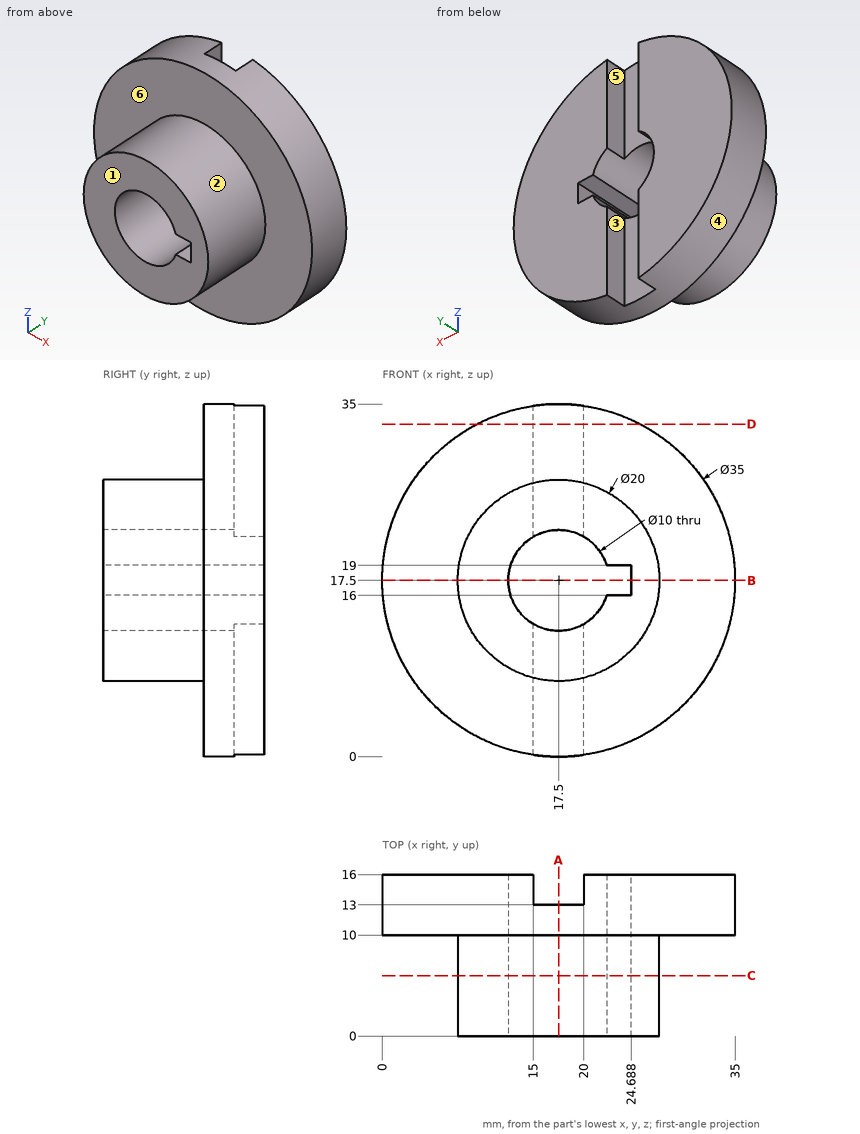
Verification items for this drawing (mm, ordinates from the low corner). A direction names the side the tool comes from. Coordinates: 2 decimals unless noted, no trailing zeros. Loops run counter-clockwise (first coordinate to the right, second up) from the corner with the lowest first, then second, coordinate; pieces in that order, holes last. Notation, with made-up numbers: (-9.5, -30.5) - (34.5, -30.5) arc R32 cw to (34.5, 2.5) - close; hole circle Ø2 at (-2.75, 70). An arc over 180 degrees is marked (long way). Use one line per item in the form item = value. Start each with the question number.
Item 1: Thickness scan on probe 1 along X at (y, z) = (5.75, 17.5); probe 2 along Z at (x, y) = (17.5, 12.75); probe 3 along Z at (x, y) = (17.5, 5.5). Record the ranges inside material, lowest first.
Item 2: Gauge pin test, flat ends, axial feed: pin 1 (2 mm diameter, centred on y = 2, z = 22, fed in from -X); pin 2 (1.5 mm diameter, centred on x = 17.5, z = 8.5, fed in from +Y); pin 3 (1.9 mm diameter, centred on x = 23.5, y = 4, fed in from +Z). Record the tip position at first contact, or that the pin passes through.
Item 3: Tool access check on the marked faces 1, 2 and 3. Record the directions out of +Z, -Z, +X, -X, +Y, -Y that give a thin tool (end or side, any length) a straight path to the whole face; none if there is none.
Item 4: Section check D-D, the plane z = 33. Enter the section's corners in (x, y).
Item 5: Mould release check, pull along X, two halves, no side actions. Record for the marked faces 4, 5 and 6: +X half, -X half, draft (parallel to the pull), parting line (faces both ways), or undercut.
Item 6: Section check A-A, the plane x = 17.5. Enter the section's corners in (y, z).
Item 7: Section check B-B, the plane z = 17.5. Enter the section's corners in (x, y), and give its area (3 significant figures).
Item 8: Section check C-C, the plane y = 6. Enter the section's corners in (x, z).
Computed:
q1.probe_1 = 7.5 to 12.5, 24.69 to 27.5
q1.probe_2 = 0 to 12.5, 22.5 to 35
q1.probe_3 = 7.5 to 12.5, 22.5 to 27.5
q2.pin_1 = 8.13
q2.pin_2 = 13
q2.pin_3 = 26.13
q3.face_1 = +Z, -Z, +X, -X, -Y
q3.face_2 = -Y
q3.face_3 = +Z, -Z, +Y
q4.outline = (9.38, 10) - (25.62, 10) - (25.62, 16) - (20, 16) - (20, 13) - (15, 13) - (15, 16) - (9.38, 16) - close
q5.face_4 = parting line
q5.face_5 = undercut
q5.face_6 = draft
q6.outline = (0, 7.5) - (10, 7.5) - (10, 0) - (13, 0) - (13, 12.5) - (0, 12.5) - close; (0, 22.5) - (13, 22.5) - (13, 35) - (10, 35) - (10, 27.5) - (0, 27.5) - close
q7.outline = (0, 10) - (7.5, 10) - (7.5, 0) - (12.5, 0) - (12.5, 16) - (0, 16) - close; (24.69, 0) - (27.5, 0) - (27.5, 10) - (35, 10) - (35, 16) - (24.69, 16) - close
q7.area = 215 mm2
q8.outline = circle Ø20 at (17.5, 17.5); hole (22.27, 16) - (24.69, 16) - (24.69, 19) - (22.27, 19) arc R5 ccw (long way) to start
